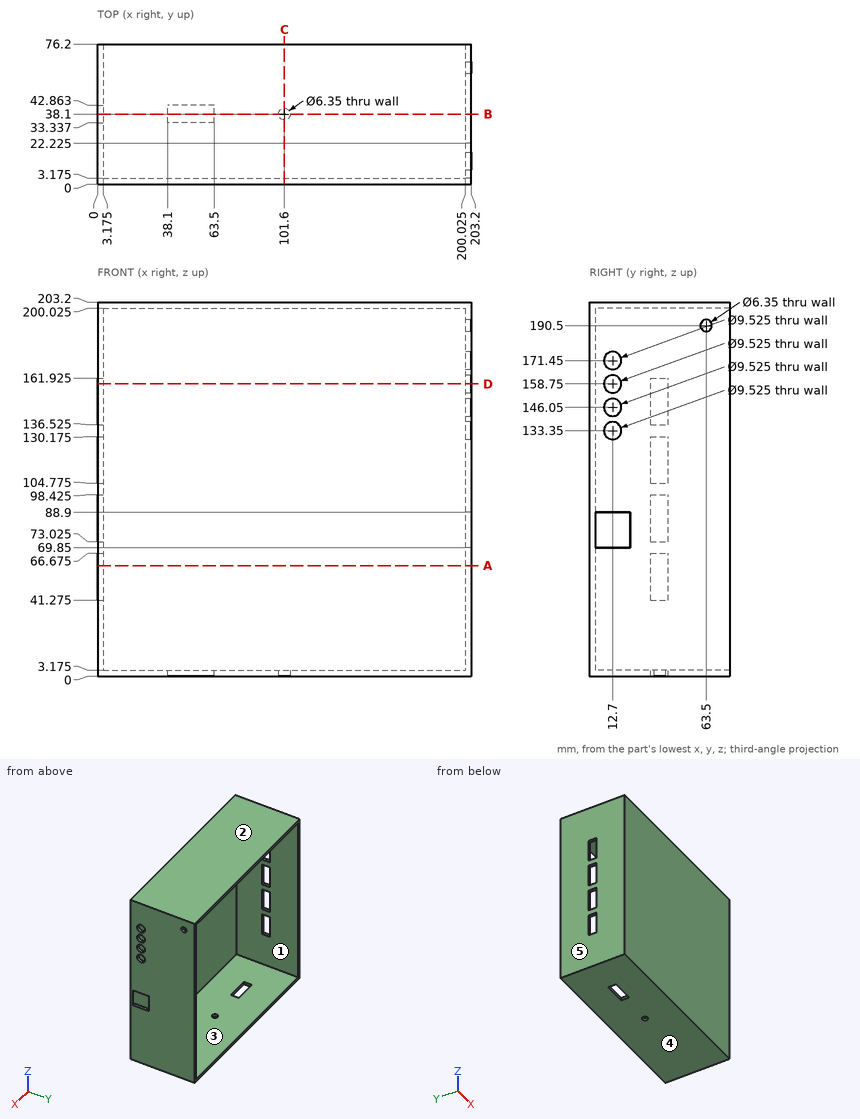
Here's the drawing with two shaded views (mm, measured from the low corner). I have some questions. A direction names the side the tool comes from. Round coordinates to 2 decimals unless told otherwise and drop trailing zeros. Loops run counter-clockwise (first coordinate to the right, second up) from the corner with the lowest first, then second, coordinate; pieces in that order, holes last.
1. Suppose I cut it at C-C, the plane x = 101.6. Please give me the cut outline in (y, z) (1 decimal), and give its area (3 significant figures).
Answers:
outline: (0, 0) - (34.9, 0) - (34.9, 3.2) - (3.2, 3.2) - (3.2, 200) - (76.2, 200) - (76.2, 203.2) - (0, 203.2) - close; (41.3, 0) - (76.2, 0) - (76.2, 3.2) - (41.3, 3.2) - close
area: 1,090 mm2
2. Suppose I cut it at A-A, the plane z = 60. Please give me the cut outline in (x, y) (1 decimal).
Answers:
outline: (0, 0) - (203.2, 0) - (203.2, 76.2) - (200, 76.2) - (200, 3.2) - (3.2, 3.2) - (3.2, 33.3) - (0, 33.3) - close; (0, 42.9) - (3.2, 42.9) - (3.2, 76.2) - (0, 76.2) - close
3. For the marked faces 1 and 2, which set-ups out of +Z, -Z, +X, -X, +Y, -Y let a thin tool reach every point of the face, with its end or its side?
Answers:
face 1: +Y
face 2: +Z, +X, -X, +Y, -Y
4. Thinking about a two-plate mould opening in X: for the marked faces 3, 4 and 5, which applies, released by +X, released by -X, zero draft, split by the parting line, or undercut?
Answers:
face 3: undercut
face 4: zero draft
face 5: released by -X
5. If I drill on probe 1 along Z at (x, y) = (201, 12); probe 2 along X at (y, z) = (11.5, 24) (1 decimal); probe 3 along Y at (x, z) = (200.7, 190.5) (1 decimal), over which ranges is the centre line in solid material (lowest first)?
Answers:
probe 1: z = 0 to 69.85, 88.9 to 128.64, 138.06 to 141.34, 150.76 to 154.04, 163.46 to 166.74, 176.16 to 203.2
probe 2: x = 0 to 3.2, 200 to 203.2
probe 3: y = 0 to 60.3, 66.7 to 76.2
6. Suppose I cut it at B-B, the plane y = 38.1. Give the number of separate pieces and of enclosed holes in the cut face, and give its area (3 significant figures).
Answers:
separate pieces: 6
enclosed holes: 0
area: 2,120 mm2
7. Will these pins go through, and if not, where does the flat tip stop? pin 1 (1.6 mm diameter, centred on x = 1.5, z = 119, fed in from -Y); pin 2 (6 mm diameter, centred on x = 67.5, z = 171, fed in from +Y) (1 decimal).
Answers:
pin 1: stops at y = 0
pin 2: stops at y = 3.2
8. Suppose I cut it at D-D, the plane z = 158.75. Please give me the cut outline in (x, y) (1 decimal).
Answers:
outline: (0, 0) - (203.2, 0) - (203.2, 7.9) - (200, 7.9) - (200, 3.2) - (3.2, 3.2) - (3.2, 33.3) - (0, 33.3) - close; (0, 42.9) - (3.2, 42.9) - (3.2, 76.2) - (0, 76.2) - close; (200, 17.5) - (203.2, 17.5) - (203.2, 76.2) - (200, 76.2) - close
